from build123d import *
from OCP.BRepFilletAPI import BRepFilletAPI_MakeChamfer

# Parameters (mm, degrees)
BOSS_EXTRUDE1_DEPTH = 6
FILLET1_R           = 2.54
SKETCH2_W           = 3.1242
SKETCH2_H           = 8.001
CUT_EXTRUDE1_DEPTH  = 18.538679192
CHAMFER1_SIZE       = 0.381
CHAMFER1_SIZE2      = 2.710955864
FILLET2_R           = 0.508


with BuildPart() as part:
    # Sketch1 → Boss-Extrude1 (new body)
    with BuildSketch(Plane.XY):
        Polygon((0, 0), (-8.167456121, 8.167456121), (-8.167456121, 8.980256121), (-4.718728061, 8.980256121), (-4.718728061, 14.314256121), (2.901271939, 14.314256121), (2.901271939, 8.980256121), (6.35, 8.980256121), (6.35, -8.980256121), (-8.167456121, -8.980256121), (-8.167456121, -8.167456121), align=None)
    extrude(amount=BOSS_EXTRUDE1_DEPTH)

    # Fillet1
    fillet1_edges = [part.edges().sort_by_distance(p)[0] for p in [
        (6.35, -8.980256121, 3),
    ]]
    fillet(fillet1_edges, radius=FILLET1_R)

    # Sketch2 → Cut-Extrude1 (cut, through all)
    with BuildSketch(Plane.XY.offset(6)):
        with Locations((-0.908728061, 10.313756121)):
            Rectangle(SKETCH2_W, SKETCH2_H)
    extrude(amount=-CUT_EXTRUDE1_DEPTH, mode=Mode.SUBTRACT)

    # Chamfer1: one chamfer whose edges measure the first distance from different faces: ONE call of the kernel's chamfer builder (chamfer() names one face for all edges)
    chamfer1_edges_1 = [part.edges().sort_by_distance(p)[0] for p in [
        (-2.470828061, 14.314256121, 3),
    ]]
    chamfer1_side_1 = [part.faces().sort_by_distance(p)[0] for p in [
        (-3.594778061, 14.314256121, 3),
    ]]
    chamfer1_edges_2 = [part.edges().sort_by_distance(p)[0] for p in [
        (0.653371939, 14.314256121, 3),
    ]]
    chamfer1_side_2 = [part.faces().sort_by_distance(p)[0] for p in [
        (1.777321939, 14.314256121, 3),
    ]]
    chamfer1 = BRepFilletAPI_MakeChamfer(part.part.solid().wrapped)
    for e in chamfer1_edges_1:
        chamfer1.Add(CHAMFER1_SIZE, CHAMFER1_SIZE2, e.wrapped, chamfer1_side_1[0].wrapped)  # the first distance lies on this face
    for e in chamfer1_edges_2:
        chamfer1.Add(CHAMFER1_SIZE, CHAMFER1_SIZE2, e.wrapped, chamfer1_side_2[0].wrapped)  # the first distance lies on this face
    add(Compound.cast(chamfer1.Shape()), mode=Mode.REPLACE)

    # Fillet2
    fillet2_edges = [part.edges().sort_by_distance(p)[0] for p in [
        (-2.470828061, 6.313256121, 3),
        (0.653371939, 6.313256121, 3),
    ]]
    fillet(fillet2_edges, radius=FILLET2_R)


solid = part.part
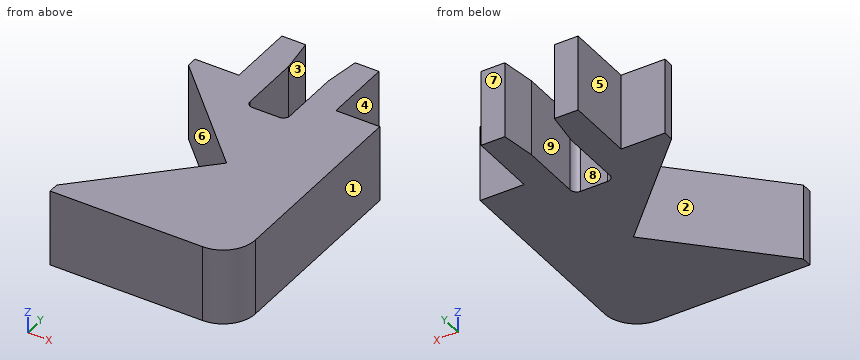
The listing builds one solid part. Answer for the finished solid, in the listing's coordinates (mm). Face numbers are marked on the shaded views. A direction names the side the tool comes from. Give positions to 0.01 mm unless a question says otherwise; leave off trailing zeros. Write each loop counter-clockwise with the first axis right and the second up, starting at its lowest first coordinate (ties: lowest second). Pieces come first, ordered by that corner, then holes.
1) Section C-C (z = 5.3) is taken. Write down the section's boundary in (x, y), and give its area (3 significant figures).
2) Find the intervals of material crossed by L1, parallel to X at y = 11, z = 4.95; L2, parallel to Y at x = -0.5, z = 1.95; L3, parallel to Y at x = -3.5, z = 3.25, in increasing order.
3) Section A-A (y = 8.75) is taken. Write down the section's boundary in (x, z), and give its area (3 significant figures).
4) Section D-D (y = 5.75) is taken. Write down the section's boundary in (x, z), and give its area (3 significant figures).
5) Given P1, Ø2.5, axis at y = 12, z = 2, coming from the -X side; P2, Ø1.7, axis at x = -1, z = 4.5, coming from the +Y side; P3, Ø1.5, axis at x = -5.5, z = 2.5, coming from the +Y side, each flat-ended and moving along its own axis, determine where each tip first touches the part or whether it passes through.
6) A tool of negligible diameter and unlimited length cuts with its end or side. For the marked faces 1, 2, 3, 4 and 5, from which of +Z, -Z, +X, -X, +Y, -Y can it reach the whole face along a straight path? Write none if from no direction.
7) Section B-B (x = -5) is taken. Write down the section's boundary in (y, z), and give its area (3 significant figures).
8) For a pull along X with two mould halves and no side action, classify the marked faces 6, 7, 8 and 9 as pulls with the +X half, pulls with the -X half, needs draft (parallel to the pull), parting line crosses it, or undercut.
Response:
1. outline: (-8.17, -8.98) - (3.81, -8.98) arc R2.54 ccw to (6.35, -6.44) - (6.35, 8.98) - (2.9, 8.98) - (2.9, 14.31) - (1.03, 14.31) - (0.65, 11.6) - (0.65, 6.82) arc R0.51 cw to (0.15, 6.31) - (-1.96, 6.31) arc R0.51 cw to (-2.47, 6.82) - (-2.47, 11.6) - (-2.85, 14.31) - (-4.72, 14.31) - (-4.72, 8.98) - (-8.17, 8.98) - (-8.17, 8.17) - (0, 0) - (-8.17, -8.17) - close
1. area: 207 mm2
2. L1: x = -4.72 to -2.47, 0.65 to 2.9
2. L2: y = -8.98 to -0.5, 0.5 to 6.31
2. L3: y = -8.98 to -3.5, 3.5 to 14.31
3. outline: (-8.17, 0) - (-2.47, 0) - (-2.47, 6) - (-8.17, 6) - close; (0.65, 0) - (6.35, 0) - (6.35, 6) - (0.65, 6) - close
3. area: 68.4 mm2
4. outline: (-5.75, 0) - (6.35, 0) - (6.35, 6) - (-5.75, 6) - close
4. area: 72.6 mm2
5. P1: stops at x = -4.72
5. P2: stops at y = 6.31
5. P3: stops at y = 8.98
6. face 1: +Z, -Z, +X, +Y, -Y
6. face 2: +Z, -Z, -X
6. face 3: +Z, -Z, +Y
6. face 4: +Z, -Z, +X, +Y
6. face 5: +Z, -Z, -X, +Y
7. outline: (-8.98, 0) - (-5, 0) - (-5, 6) - (-8.98, 6) - close; (5, 0) - (8.98, 0) - (8.98, 6) - (5, 6) - close
7. area: 47.8 mm2
8. face 6: pulls with the -X half
8. face 7: needs draft
8. face 8: undercut
8. face 9: undercut
